The drawing under review shows one solid part. Ordinate dimensions are in mm from its lowest x, y, z. Give positions to 0.01 mm unless a question says otherwise; leave off trailing zeros. Write each loop counter-clockwise with the first axis right and the second up, starting at its lowest first coordinate (ties: lowest second). Pieces come first, ordered by that corner, then holes. Notation, with made-up numbers: (28.5, 46) - (49.5, 46) arc R21 ccw to (49.5, 81) - close; hole circle Ø8 at (33.25, 58). An arc over 180 degrees is marked (long way). Write item = value, one per line.
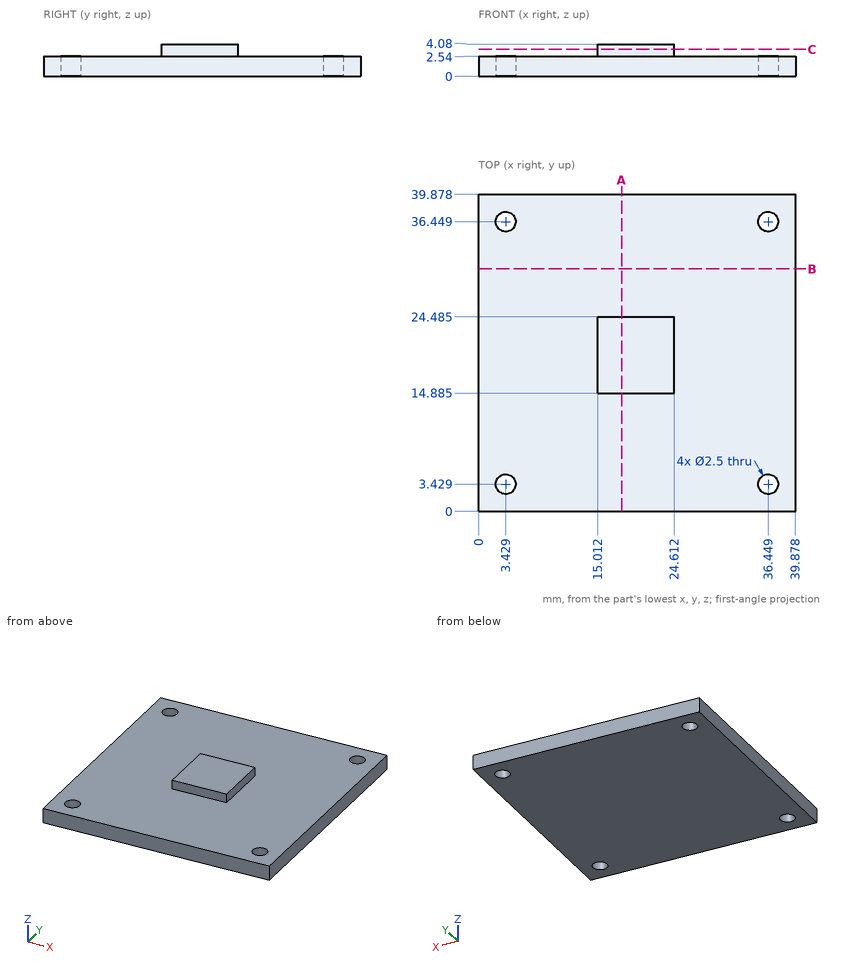
1. Take a section at C-C on z = 3.4. Give the boundary of the cut face in (x, y) (3 decimals).
Findings below:
outline = (15.012, 14.885) - (24.612, 14.885) - (24.612, 24.485) - (15.012, 24.485) - close
2. For line 1 (Y direction, x = 3, z = 1.8) (3 decimals); line 2 (X direction, y = 36, z = 0.35); line 3 (Z direction, x = 26, y = 32), list the stretches that pass through material, from the lowest coordinate up. Write a range as from..to.
Findings below:
line_1 = 0..2.255, 4.603..35.275, 37.623..39.878
line_2 = 0..2.26, 4.6..35.28, 37.62..39.88
line_3 = 0..2.54
3. Take a section at A-A on x = 18. Give the boundary of the cut face in (y, z) (3 decimals).
Findings below:
outline = (0, 0) - (39.878, 0) - (39.878, 2.54) - (24.485, 2.54) - (24.485, 4.08) - (14.885, 4.08) - (14.885, 2.54) - (0, 2.54) - close
4. Insertion check: P1, Ø3, axis at x = 36.45, y = 36.45, coming from the +Z side; P2, Ø0.8, axis at x = 20, z = 3.5, coming from the -Y side (3 decimals); P3, Ø0.5, axis at y = 18, z = 3.5, coming from the -X side. Each pin has a flat end and moves straight along its axis. Give the tip position at first contact, or say it passes through.
Findings below:
P1 = 2.54
P2 = 14.885
P3 = 15.01
5. Take a section at B-B on y = 30.5. Give the boundary of the cut face in (x, z), and give its area (3 significant figures).
Findings below:
outline = (0, 0) - (39.88, 0) - (39.88, 2.54) - (0, 2.54) - close
area = 101 mm²
